Check sheet for the modelled part. Datum: model origin and axes. Units: mm. A direction names the side the tool comes from. Round coordinates to 2 decimals unless told otherwise and drop trailing zeros. Loops run counter-clockwise (first coordinate to the right, second up) from the corner with the lowest first, then second, coordinate; pieces in that order, holes last. Notation, with made-up numbers: (18, 33) - (64, 33) arc R19 cw to (64, 55) - close; hole circle Ø4 at (81, -13.75). An arc over 180 degrees is marked (long way). Answer in a Markdown table with one row per item. Add a question column.
(1) Access from +Z, -Z, +X, -X, +Y, -Y to the whole of each face (thin tool, end or side, straight path). Record for faces 3 (the flat face through (3, 16, -1)), 4 (the flat face through (-4, 0, 4)).
(2) Mould release check, pull along X, two halves, no side actions. Record for faces 1 (the flat face through (0, 24, 4)), 2 (the cylindrical face through (0.9, 19.8, 2.86)): +X half, -X half, draft (parallel to the pull), parting line (faces both ways), or undercut.
(3) Cross-section at A-A on y = 19.5. Enter the section's corners in (x, z).
(4) Gauge pin test, flat ends, axial feed: pin 1 (1.5 mm diameter, centred on x = -2, z = 3, fed in from -Y); pin 2 (5 mm diameter, centred on x = 0, z = 0, fed in from -Y); pin 3 (3 mm diameter, centred on y = 21, z = 2, fed in from +X). Record the tip position at first contact, or that the pin passes through.
(5) Cross-section at D-D on y = 2.75. Enter the section's corners in (x, z).
(6) Thickness scan on line 1 along X through (y, z) = (2.25, 0); line 2 along X through (y, z) = (19.25, 0); line 3 along Y through (x, z) = (1, 7.5). Record the ranges inside material, lowest first.
(7) Cross-section at B-B on z = 0. Count the separate pieces of the cut face and the enclosed holes in it, then the cut area to 3 significant figures.
from build123d import *

# Parameters (mm, degrees)
SKETCH1_R           = 9
BOSS_EXTRUDE1_DEPTH = 24
SKETCH2_R           = 3
CUT_EXTRUDE1_DEPTH  = 28.166155414
SKETCH3_R           = 4
CUT_EXTRUDE2_DEPTH  = 16
CHAMFER1_SIZE       = 0.5
CUT_SWEEP2_PITCH    = 2


with BuildPart() as part:
    # Sketch1 → Boss-Extrude1 (new body)
    with BuildSketch(Plane(origin=(0, 0, 0), x_dir=(1, 0, 0), z_dir=(0, 1, 0))):
        with Locations(Location((0, 0, 0), (0, 0, 270))):
            Circle(SKETCH1_R)
    extrude(amount=BOSS_EXTRUDE1_DEPTH)

    # Sketch2 → Cut-Extrude1 (cut, through all)
    with BuildSketch(Plane(origin=(0, 24, 0), x_dir=(1, 0, 0), z_dir=(0, 1, 0))):
        with Locations(Location((0, 0, 0), (0, 0, 270))):
            Circle(SKETCH2_R)
    extrude(amount=-CUT_EXTRUDE1_DEPTH, mode=Mode.SUBTRACT)

    # Sketch3 → Cut-Extrude2 (cut)
    with BuildSketch(Plane.XZ):
        with Locations(Location((0, 0, 0), (0, 0, 270))):
            Circle(SKETCH3_R)
    extrude(amount=-CUT_EXTRUDE2_DEPTH, mode=Mode.SUBTRACT)

    # Chamfer1
    chamfer1_edges = [part.edges().sort_by_distance(p)[0] for p in [
        (0, 0, 4),
        (0, 0, -9),
        (0, 24, -9),
        (0, 24, -3),
    ]]
    chamfer(chamfer1_edges, length=CHAMFER1_SIZE)

    # Cut-Sweep2: the profile of Sketch8 profile screwed along a left-hand helix of 5 turns, 10 arcs to a turn; built about Z, then put on its axis
    cut_sweep2_z = Axis((0, 0, 0), (0, 0, 1))
    cut_sweep2_corners = [(9, 0, 0), (3.9997, 0, 0), (3.9997, 0, 0.5), (9, 0, 0.5)]
    with BuildLine(mode=Mode.PRIVATE) as cut_sweep2_profile:
        Line(cut_sweep2_corners[0], cut_sweep2_corners[1])
        Line(cut_sweep2_corners[1], cut_sweep2_corners[2])
        Line(cut_sweep2_corners[2], cut_sweep2_corners[3])
        Line(cut_sweep2_corners[3], cut_sweep2_corners[0])
    cut_sweep2_cap = Face(cut_sweep2_profile.wire())
    cut_sweep2_turn_angles = [0, -18, -36, -54, -72, -90, -108, -126, -144, -162, -180, -198, -216, -234, -252, -270, -288, -306, -324, -342, -360]
    cut_sweep2_turn_weights = [1, 0.9510565162951535, 1, 0.9510565162951535, 1, 0.9510565162951535, 1, 0.9510565162951535, 1, 0.9510565162951535, 1, 0.9510565162951535, 1, 0.9510565162951535, 1, 0.9510565162951535, 1, 0.9510565162951535, 1, 0.9510565162951535, 1]
    cut_sweep2_turn_rails = [Edge.make_bspline([Vector(p[0], p[1], 0).rotate(cut_sweep2_z, cut_sweep2_turn_angles[k]) / cut_sweep2_turn_weights[k] + Vector(0, 0, p[2] + -CUT_SWEEP2_PITCH * cut_sweep2_turn_angles[k] / 360) for k in range(21)], [0, 0, 0, 1, 1, 2, 2, 3, 3, 4, 4, 5, 5, 6, 6, 7, 7, 8, 8, 9, 9, 10, 10, 10], 2, cut_sweep2_turn_weights) for p in cut_sweep2_corners]
    cut_sweep2_turn_sides = [Face.make_surface_from_curves(cut_sweep2_turn_rails[p[0]], cut_sweep2_turn_rails[p[1]]) for p in [(0, 1), (1, 2), (2, 3), (3, 0)]]
    cut_sweep2 = Plane(origin=(0, 16, 0), x_dir=(0, 0, -1), z_dir=(0, -1, 0)) * Solid(Shell([*[p.moved(Location((0, 0, CUT_SWEEP2_PITCH * i))) for i in range(5) for p in cut_sweep2_turn_sides], cut_sweep2_cap, cut_sweep2_cap.rotate(cut_sweep2_z, -1800).moved(Location((0, 0, -CUT_SWEEP2_PITCH * -1800 / 360)))]))
    add(cut_sweep2, mode=Mode.SUBTRACT)


solid = part.part
Answers:
| question | item | result |
|---|---|---|
| 1 | face 3 | -Y |
| 1 | face 4 | +Z, -Z, +X, -X, -Y |
| 2 | face 1 | draft |
| 2 | face 2 | undercut |
| 3 | outline | circle Ø18 at (0, 0); hole circle Ø6 at (0, 0) |
| 4 | pin 1 | stops at y = 0.14 |
| 4 | pin 2 | passes through |
| 4 | pin 3 | stops at x = 8.99 |
| 5 | outline | circle Ø18 at (0, 0); hole circle Ø8 at (0, 0) |
| 6 | line 1 | x = -9 to -4, 4 to 9 |
| 6 | line 2 | x = -9 to -3, 3 to 9 |
| 6 | line 3 | y = 0 to 6.46, 6.96 to 8.46, 8.96 to 10.46, 10.96 to 12.46, 12.96 to 14.46, 14.96 to 24 |
| 7 | separate pieces | 12 |
| 7 | enclosed holes | 0 |
| 7 | area | 230 mm^2 |
